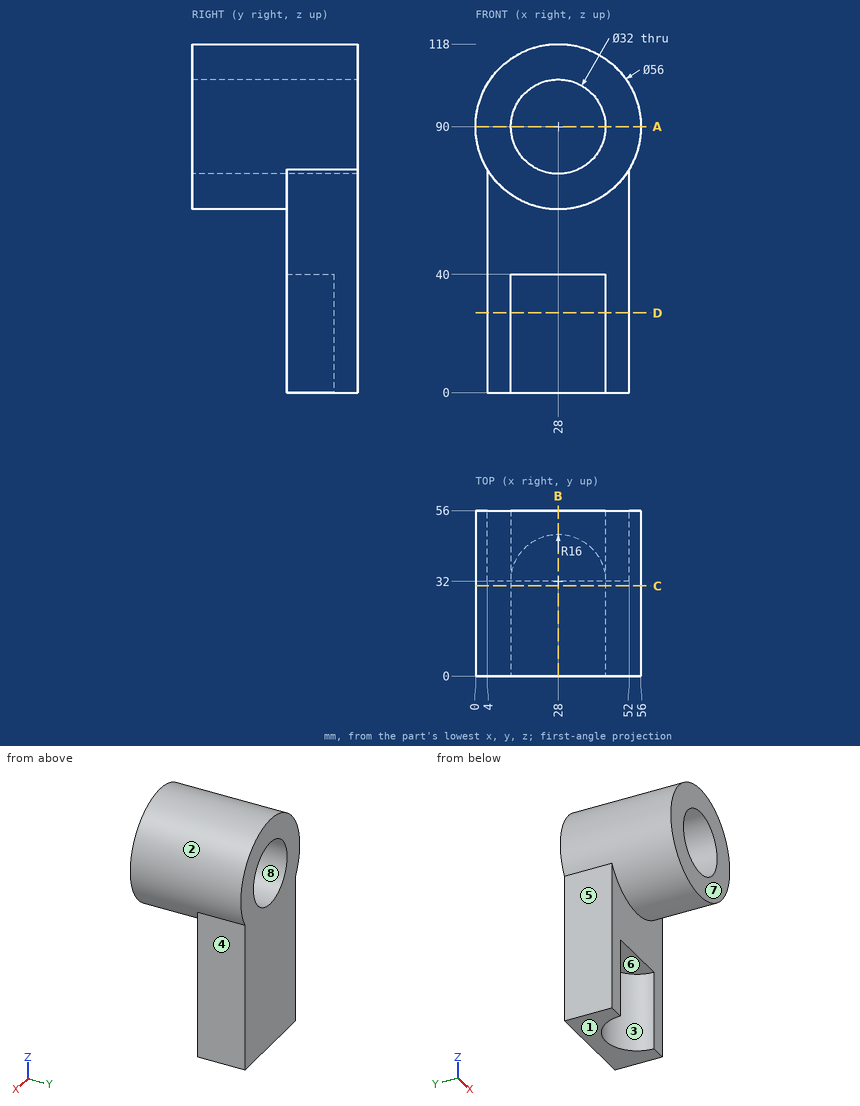
The figure shows three views and two pictorial views of one solid part (mm, origin at its lowest corner). Answer the questions. A direction names the side the tool comes from. Give positions to 0.01 mm unless a question says otherwise; leave off trailing zeros. Write each loop counter-clockwise with the first axis right and the second up, starting at its lowest first coordinate (ties: lowest second). Pieces come first, ordered by that corner, then holes. Notation, with made-up numbers: M -37,29.25 L 22,29.25 A20 cw 22,50.25 Z; hole C 26,44 d1. An arc over 180 degrees is marked long. Write each question's results on one line, items separated by ' | '.
Q1. For a pull along X with two mould halves and no side action, classify the marked faces 1, 2 and 3 as released by +X, released by -X, zero draft, split by the parting line, or undercut.
Output values:
face 1: zero draft | face 2: split by the parting line | face 3: undercut
Q2. Section D-D, the plane z = 27 is taken. Write down the section's boundary in (x, y).
Output values:
outline: M 4,32 L 12,32 A16 cw 44,32 L 52,32 L 52,56 L 4,56 Z
Q3. Section C-C, the plane y = 30.5 is taken. Write down the section's boundary in (x, z), then the cut area to 3 significant figures.
Output values:
outline: C 28,90 d56; hole C 28,90 d32 | area: 1,660 mm2
Q4. Section B-B, the plane x = 28 is taken. Write down the section's boundary in (y, z), then the cut area to 3 significant figures.
Output values:
outline: M 0,62 L 32,62 L 32,40 L 48,40 L 48,0 L 56,0 L 56,74 L 0,74 Z; M 0,106 L 56,106 L 56,118 L 0,118 Z | area: 2,190 mm2
Q5. Flat-ended cylindrical pins translate along their axes: P1, Ø19, axis at y = 49, z = 47.5, coming from the -X side; P2, Ø14.5, axis at x = 35, z = 34, coming from the -Y side; P3, Ø2, axis at x = 47, y = 23.5, coming from the +Z side. Find the tip coordinate at first contact, or state that the pin passes through.
Output values:
P1: x = 4 | P2: y = 32 | P3: z = 111.45
Q6. Consider L1, parallel to X at y = 41, z = 90; L2, parallel to Y at x = 28, z = 27; L3, parallel to X at y = 25, z = 84.5. Determine where each line is inside the solid, lowest interval first. Write a range as from..to.
Output values:
L1: 0..12, 44..56 | L2: 48..56 | L3: 0.55..12.98, 43.02..55.45
Q7. A tool of negligible diameter and unlimited length cuts with its end or side. For the marked faces 4, 5, 6, 7 and 8, from which of +Z, -Z, +X, -X, +Y, -Y can it reach the whole face along a straight path? Write none if from no direction.
Output values:
face 4: -Z, +X, +Y, -Y | face 5: -Z, -X, +Y, -Y | face 6: -Z, -Y | face 7: +Z, -Z, +X, -X, -Y | face 8: +Y, -Y
Q8. Section A-A, the plane z = 90 is taken. Write down the section's boundary in (x, y).
Output values:
outline: M 0,0 L 12,0 L 12,56 L 0,56 Z; M 44,0 L 56,0 L 56,56 L 44,56 Z
